Can you work these out from the model? Positions are in its coordinate system, mm. A direction names the side the tool comes from. Round coordinates to 2 decimals unless told otherwise and drop trailing zeros. Write each loop counter-clockwise with the first axis right and the second up, starting at its lowest first coordinate (ties: lowest second). Pieces come first, ordered by that corner, then holes. Notation, with made-up numbers: M 85,-1 L 125,-1 A24 cw 125,21 Z; hole C -17.5,28.25 d1. An arc over 180 degrees is marked long. Answer as a JSON object with one key per item and string values. Group by question number.
1) Suppose I cut it at B-B, the plane z = 0. Write out the boundary of the cut face in (x, y), and give its area (3 significant figures).
2) If we mould it in two halves opening along X, with no side actions, what happens to faces 3 (the flat face through (-5, 0, -35)), 4 (the cylindrical face through (-320, 3, 50))? For each: +X half, -X half, draft (parallel to the pull), parting line (faces both ways), or undercut.
3) Suppose I cut it at D-D, the plane x = 0. Write out the boundary of the cut face in (y, z), and give its area (3 significant figures).
4) I'm going to push a flat-ended pin straight in: pin 1 Ø12 at (x, z) = (50, 100) entering from -Y. Where does the tip first touch, or does it pass through?
5) Please list where these lines run through material, in increasing order: L1, parallel to X at y = 5, z = 0; L2, parallel to X at y = 2, z = 14; L3, parallel to Z at x = -6, y = 0.75. Write a range as [from, to].
6) On a 3-axis mill with a long thin cutter (end or side, diameter ignored), from which of +Z, -Z, +X, -X, +Y, -Y can I reach the whole of each face in a straight line? I mean faces 1 (the flat face through (-5, 6.35, -35)), 2 (the cylindrical face through (320, 3, -50)). Say none if no direction works.
7) Suppose I cut it at A-A, the plane x = -320. Write out the boundary of the cut face in (y, z), and give its area (3 significant figures).
8) Suppose I cut it at C-C, the plane y = 5.25. Write out the boundary of the cut face in (x, z), and give its area (3 significant figures).
from build123d import *

# Parameters (mm, degrees)
SKETCH1_W         = 740
SKETCH1_H         = 293
BASE_DEPTH        = 6.35
HANDLES_DEPTH     = 398.998206654
SKETCH3_R         = 20
CAMERA_HOLE_DEPTH = 398.998206654


with BuildPart() as part:
    # Sketch1 → Base (new body)
    with BuildSketch(Plane(origin=(0, 0, 0), x_dir=(1, 0, 0), z_dir=(0, 1, 0))):
        Rectangle(SKETCH1_W, SKETCH1_H)
    extrude(amount=BASE_DEPTH)

    # Sketch2 → Handles (cut, through all)
    with BuildSketch(Plane(origin=(0, 6.35, 0), x_dir=(1, 0, 0), z_dir=(0, 1, 0))):
        with BuildLine():
            Line((-335, -35), (-335, 35))
            ThreePointArc((-335, 35), (-320, 50), (-305, 35))
            Line((-305, 35), (-305, -35))
            ThreePointArc((-305, -35), (-320, -50), (-335, -35))
        make_face()
        with BuildLine():
            Line((335, -35), (335, 35))
            ThreePointArc((335, 35), (320, 50), (305, 35))
            Line((305, 35), (305, -35))
            ThreePointArc((305, -35), (320, -50), (335, -35))
        make_face()
    extrude(amount=-HANDLES_DEPTH, mode=Mode.SUBTRACT)

    # Sketch3 → Camera Hole (cut, through all)
    with BuildSketch(Plane(origin=(0, 6.35, 0), x_dir=(1, 0, 0), z_dir=(0, 1, 0))):
        with Locations(Location((0, 0, 0), (0, 0, 270))):
            Circle(SKETCH3_R)
    extrude(amount=-CAMERA_HOLE_DEPTH, mode=Mode.SUBTRACT)


solid = part.part
Results:
{
 "1": {"outline": "M -370,0 L -335,0 L -335,6.35 L -370,6.35 Z; M -305,0 L -20,0 L -20,6.35 L -305,6.35 Z; M 20,0 L 305,0 L 305,6.35 L 20,6.35 Z; M 335,0 L 370,0 L 370,6.35 L 335,6.35 Z", "area": "4,060 mm^2"},
 "2": {"face 3": "draft", "face 4": "undercut"},
 "3": {"outline": "M 0,-146.5 L 6.35,-146.5 L 6.35,-20 L 0,-20 Z; M 0,20 L 6.35,20 L 6.35,146.5 L 0,146.5 Z", "area": "1,610 mm^2"},
 "4": {"pin 1": "y = 0"},
 "5": {"L1": "[-370, -335], [-305, -20], [20, 305], [335, 370]", "L2": "[-370, -335], [-305, -14.28], [14.28, 305], [335, 370]", "L3": "[-146.5, -19.08], [19.08, 146.5]"},
 "6": {"face 1": "+Z, -Z, +X, -X, +Y", "face 2": "+Y, -Y"},
 "7": {"outline": "M 0,-146.5 L 6.35,-146.5 L 6.35,-50 L 0,-50 Z; M 0,50 L 6.35,50 L 6.35,146.5 L 0,146.5 Z", "area": "1,230 mm^2"},
 "8": {"outline": "M -370,-146.5 L 370,-146.5 L 370,146.5 L -370,146.5 Z; hole M -335,-35 A15 ccw -305,-35 L -305,35 A15 ccw -335,35 Z; hole C 0,0 d40; hole M 305,-35 A15 ccw 335,-35 L 335,35 A15 ccw 305,35 Z", "area": "210,000 mm^2"}
}
